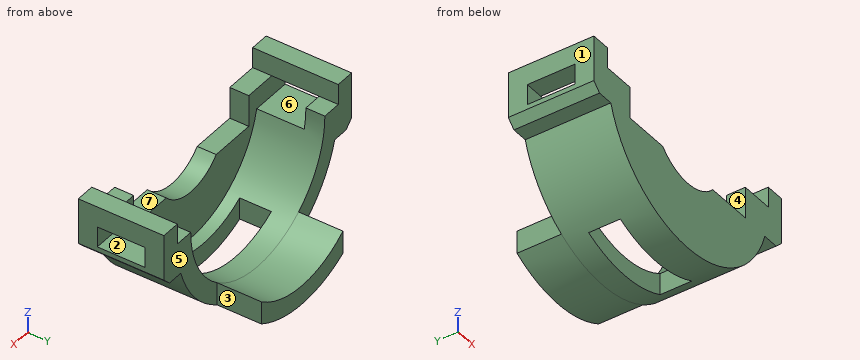
from build123d import *

# Parameters (mm, degrees)
SKETCH1_W                 = 6
SKETCH1_H                 = 1.2
SKETCH1_W_2               = 1.2
SKETCH1_H_2               = 4.2
REVOLVE1_ANGLE            = 180
REVOLVE2_START            = 4.2
REVOLVE2_DEPTH            = 2.8
SKETCH4_W                 = 6.4
SKETCH4_H                 = 2
CUT_EXTRUDE1_DEPTH        = 10
CUT_EXTRUDE2_DEPTH        = 10
BOSS_EXTRUDE6_DEPTH       = 1.2
SKETCH12_W                = 2
SKETCH12_H                = 2.1
BOSS_EXTRUDE15_DEPTH      = 5.4
SKETCH13_W                = 1.3
SKETCH13_H                = 3
CUT_EXTRUDE4_DEPTH        = 4
CUT_EXTRUDE5_DEPTH        = 4
CUT_EXTRUDE5_DEPTH_BACK   = 4
SKETCH14_W                = 1.3
SKETCH14_H                = 3
BOSS_EXTRUDE16_DEPTH      = 2.3
BOSS_EXTRUDE16_DEPTH_BACK = 0.1
SKETCH15_W                = 3.4
SKETCH15_H                = 5.4
SKETCH15_W_2              = 1.3
SKETCH15_H_2              = 3
SKETCH16_W                = 1.2
SKETCH16_H                = 1.3
CUT_EXTRUDE6_DEPTH        = 13.310970717
CHAMFER2_SIZE             = 0.5


# Read off the part's stored shape, not the designer's step: Revolve2
with BuildPart() as part:
    # Sketch1 → Revolve1 (revolve)
    with BuildSketch(Plane.XY):
        with Locations((3, -0.6)):
            Rectangle(SKETCH1_W, SKETCH1_H)
        with Locations((6.6, -0.6)):
            Rectangle(SKETCH1_W_2, SKETCH1_H)
        with Locations((6.6, 2.1)):
            Rectangle(SKETCH1_W_2, SKETCH1_H_2)
    revolve(axis=Axis((0, -1.2, 0), (0, 1, 0)), revolution_arc=REVOLVE1_ANGLE)

    # Revolve2 outline → Revolve2 (add)
    with BuildSketch(Plane(origin=(0, 0, 0), x_dir=(1, 0, 0), z_dir=(0, 1, 0)).offset(REVOLVE2_START)):
        with BuildLine():
            ThreePointArc((3.65, 6.206246853), (0, 7.2), (-3.65, 6.206246853))
            Line((-3.65, 6.206246853), (-3.65, 4.762089877))
            ThreePointArc((-3.65, 4.762089877), (0, 6), (3.65, 4.762089877))
            Line((3.65, 4.762089877), (3.65, 6.206246853))
        make_face()
    extrude(amount=REVOLVE2_DEPTH)

    # Sketch4 → Cut-Extrude1 (cut)
    with BuildSketch(Plane.XY):
        with Locations((0, 1.8)):
            Rectangle(SKETCH4_W, SKETCH4_H)
    extrude(amount=-CUT_EXTRUDE1_DEPTH, mode=Mode.SUBTRACT)

    # Sketch5 → Cut-Extrude2 (cut)
    with BuildSketch(Plane(origin=(0, 0, 0), x_dir=(1, 0, 0), z_dir=(0, 1, 0))):
        with BuildLine():
            Line((-5.15, 2), (-5.15, 0))
            Line((-5.15, 0), (-3, 0))
            ThreePointArc((-3, 0), (-2.802517077, 1.070466269), (-2.236067977, 2))
            Line((-2.236067977, 2), (-5.15, 2))
        make_face()
        with BuildLine():
            ThreePointArc((-2.236067977, 2), (-2.802517077, 1.070466269), (-3, 0))
            Line((-3, 0), (3, 0))
            ThreePointArc((3, 0), (2.802517077, 1.070466269), (2.236067977, 2))
            Line((2.236067977, 2), (-2.236067977, 2))
        make_face()
        with BuildLine():
            Line((-5.15, 0), (-5.15, -2))
            Line((-5.15, -2), (-2.236067977, -2))
            ThreePointArc((-2.236067977, -2), (-2.802517077, -1.070466269), (-3, 0))
            Line((-3, 0), (-5.15, 0))
        make_face()
        with BuildLine():
            ThreePointArc((-3, 0), (-2.802517077, -1.070466269), (-2.236067977, -2))
            Line((-2.236067977, -2), (2.236067977, -2))
            ThreePointArc((2.236067977, -2), (2.802517077, -1.070466269), (3, 0))
            Line((3, 0), (-3, 0))
        make_face()
        with BuildLine():
            ThreePointArc((2.236067977, 2), (0, 3), (-2.236067977, 2))
            Line((-2.236067977, 2), (2.236067977, 2))
        make_face()
        with BuildLine():
            ThreePointArc((2.236067977, 2), (2.802517077, 1.070466269), (3, 0))
            Line((3, 0), (5.15, 0))
            Line((5.15, 0), (5.15, 2))
            Line((5.15, 2), (2.236067977, 2))
        make_face()
        with BuildLine():
            ThreePointArc((3, 0), (2.802517077, -1.070466269), (2.236067977, -2))
            Line((2.236067977, -2), (5.15, -2))
            Line((5.15, -2), (5.15, 0))
            Line((5.15, 0), (3, 0))
        make_face()
    extrude(amount=-CUT_EXTRUDE2_DEPTH, mode=Mode.SUBTRACT)



with BuildPart() as body_2:
    # Sketch9 → Boss-Extrude6 (new body)
    with BuildSketch(Plane(origin=(-7.2, 0, 0), x_dir=(0, 0, -1), z_dir=(1, 0, 0))):
        Polygon((2.1, -1.2), (2.1, 4.2), (0, 4.2), (0, 3), (1.3, 3), (1.3, 0), (0, 0), (0, -1.2), align=None)
        Polygon((0, 3), (0, 4.2), (-1.3, 4.2), (-1.3, -1.2), (0, -1.2), (0, 0), align=None)
    extrude(amount=-BOSS_EXTRUDE6_DEPTH)


with BuildPart() as part_1:
    add(part.part)

    add(body_2.part)  # Boss-Extrude15 merges body 2
    # Sketch12 → Boss-Extrude15 (add)
    with BuildSketch(Plane(origin=(0, 4.2, 0), x_dir=(1, 0, 0), z_dir=(0, 1, 0))):
        with Locations((-7, 1.05)):
            Rectangle(SKETCH12_W, SKETCH12_H)
    extrude(amount=-BOSS_EXTRUDE15_DEPTH)

    # Sketch13 → Cut-Extrude4 (cut)
    with BuildSketch(Plane.ZY.offset(8.4)):
        with Locations((-0.65, 1.5)):
            Rectangle(SKETCH13_W, SKETCH13_H)
    extrude(amount=-CUT_EXTRUDE4_DEPTH, mode=Mode.SUBTRACT)

    # Sketch14 → Cut-Extrude5 (cut, two sides: drawn at the far end of the back side and taken through both)
    with BuildSketch(Plane(origin=(6.1, 0, 0), x_dir=(0, 0, -1), z_dir=(1, 0, 0)).offset(-CUT_EXTRUDE5_DEPTH_BACK)):
        with Locations((0.65, 1.5)):
            Rectangle(SKETCH14_W, SKETCH14_H)
    extrude(amount=CUT_EXTRUDE5_DEPTH + CUT_EXTRUDE5_DEPTH_BACK, mode=Mode.SUBTRACT)

    # Sketch15 → Boss-Extrude16 (add, two sides: drawn at the far end of the back side and taken through both)
    with BuildSketch(Plane(origin=(6.1, 0, 0), x_dir=(0, 0, -1), z_dir=(1, 0, 0)).offset(-BOSS_EXTRUDE16_DEPTH_BACK)):
        with Locations((0.4, 1.5)):
            Rectangle(SKETCH15_W, SKETCH15_H)
        with Locations((0.65, 1.5)):
            Rectangle(SKETCH15_W_2, SKETCH15_H_2, mode=Mode.SUBTRACT)
    extrude(amount=BOSS_EXTRUDE16_DEPTH + BOSS_EXTRUDE16_DEPTH_BACK)

    # Sketch16 → Cut-Extrude6 (cut, through all)
    with BuildSketch(Plane(origin=(0, 4.2, 0), x_dir=(1, 0, 0), z_dir=(0, 1, 0))):
        with Locations((6.6, -0.65)):
            Rectangle(SKETCH16_W, SKETCH16_H)
    extrude(amount=-CUT_EXTRUDE6_DEPTH, mode=Mode.SUBTRACT)

    # Chamfer2
    chamfer2_edges = [part_1.edges().sort_by_distance(p)[0] for p in [
        (-8.4, 1.5, -2.1),
        (8.4, 1.5, -2.1),
    ]]
    chamfer(chamfer2_edges, length=CHAMFER2_SIZE)


solid = part_1.part
Build history of the part. All positions in model axes, mm. Face numbers are marked on the shaded views. A direction names the side the tool comes from. Coordinates: 2 decimals unless noted, no trailing zeros. Write each loop counter-clockwise with the first axis right and the second up, starting at its lowest first coordinate (ties: lowest second). Pieces come first, ordered by that corner, then holes. Notation, with made-up numbers: (-16, -33.75) -> (11, -33.75) arc R20 ccw to (11, -20.75) -> close; hole circle Ø10 at (69.25, 82.5). An arc over 180 degrees is marked (long way). Use CSV: the item, a comma, the result in double quotes. Start each with the question number.
Q1. Cut at D-D, the plane y = 3.75. List the corners of the cut face in (x, z).
Q2. 3-axis set-ups, long thin cutter, end or side, ignore diameter. For the marked faces 5, 6 and 7: which of +Z, -Z, +X, -X, +Y, -Y reach the whole face in a straight line?
Q3. Pull direction X, two halves, no side cores. Call the marked faces 1, 2, 3 and 4: released by +X, released by -X, zero draft, split by the parting line, or undercut.
Q4. Cut at C-C, the plane z = 0.5. List the corners of the cut face in (x, y).
Q5. Drill centre lines: probe 1 along Y at (x, z) = (-2.25, -6.75); probe 2 along X at (y, z) = (1, 0.75); probe 3 along Y at (x, z) = (2.5, -5). Where is each one in solid material? Low to high.
Q6. Cut at B-B, the plane x = 0. List the corners of the cut face in (y, z), then the cut area to 3 significant figures.
Q7. Flat gauge pins, fed straight in: pin 1 Ø3 at (x, y) = (-3, 0) entering from -Z; pin 2 Ø1 at (x, y) = (3.5, -0.5) entering from +Z; pin 3 Ø1.2 at (y, z) = (5.5, -6) entering from -X. Where does each tip first touch, or does it go through?
Q8. Cut at A-A, the plane y = 1.75. List the corners of the cut face in (x, z).
Checked values:
1,outline,"(-8.4, -1.6) -> (-7.9, -2.1) -> (-6.89, -2.1) arc R7.2 ccw to (6.89, -2.1) -> (7.9, -2.1) -> (8.4, -1.6) -> (8.4, 1.3) -> (7.2, 1.3) -> (7.2, 0) -> (6, 0) arc R6 cw to (-6, 0) -> (-7.2, 0) -> (-7.2, 1.3) -> (-8.4, 1.3) -> close"
2,face 5,"+Z, -Z, +X, +Y"
2,face 6,"+X, -X"
2,face 7,"+Z, +Y, -Y"
3,face 1,"released by -X"
3,face 2,"zero draft"
3,face 3,"released by +X"
3,face 4,"undercut"
4,outline,"(-8.4, -1.2) -> (-7.2, -1.2) -> (-7.2, 4.2) -> (-8.4, 4.2) -> close; (7.2, -1.2) -> (8.4, -1.2) -> (8.4, 4.2) -> (7.2, 4.2) -> close"
5,probe 1,"y = -1.2 to 0.8, 2.8 to 7"
5,probe 2,"x = -8.4 to -7.2, 7.2 to 8.4"
5,probe 3,"y = -1.2 to 0"
6,outline,"(-1.2, -7.2) -> (0.8, -7.2) -> (0.8, -6) -> (0, -6) -> (0, -3) -> (-1.2, -3) -> close; (2.8, -7.2) -> (7, -7.2) -> (7, -6) -> (2.8, -6) -> close"
6,area,"11.0 mm²"
7,pin 1,"stops at z = -7.04"
7,pin 2,"stops at z = -2"
7,pin 3,"stops at x = -3.65"
8,outline,"(-8.4, -1.6) -> (-7.9, -2.1) -> (-6.89, -2.1) arc R7.2 ccw to (-3.2, -6.45) -> (-3.2, -5.08) arc R6 cw to (-5.86, -1.3) -> (-8.4, -1.3) -> close; (-8.4, 0) -> (-7.2, 0) -> (-7.2, 1.3) -> (-8.4, 1.3) -> close; (3.2, -6.45) arc R7.2 ccw to (6.89, -2.1) -> (7.9, -2.1) -> (8.4, -1.6) -> (8.4, -1.3) -> (5.86, -1.3) arc R6 cw to (3.2, -5.08) -> close; (7.2, 0) -> (8.4, 0) -> (8.4, 1.3) -> (7.2, 1.3) -> close"
